```python
from build123d import *

# Parameters (mm, degrees)
F0_W     = 25
F0_H     = 25
F1_DEPTH = 50
F2_R     = 5.15
F3_DEPTH = 50.001
F5_START = -18
F4_R     = 5.15
F5_DEPTH = 32.001
F6_R     = 1
F7_SIZE  = 0.4
F8_ANGLE = 180


with BuildPart() as f1:
    # F0 (on Top) → F1 (new body)
    with BuildSketch(Plane.XY):
        Rectangle(F0_W, F0_H)
    extrude(amount=F1_DEPTH)

    # F2 (on face) → F3 (cut, through all)
    with BuildSketch(Plane.XY.offset(50)):
        Circle(F2_R)
    extrude(amount=-F3_DEPTH, mode=Mode.SUBTRACT)

    # F4 (on face) → F5 (cut)
    with BuildSketch(Plane.XY.offset(50).offset(F5_START)):
        Polygon((5.0806823689, 8.8), (-5.0806823689, 8.8), (-10.1613647377, 0), (-5.0806823689, -8.8), (5.0806823689, -8.8), (10.1613647377, 0), align=None)
        Circle(F4_R, mode=Mode.SUBTRACT)
    extrude(amount=-F5_DEPTH, mode=Mode.SUBTRACT)

    # F6
    f6_edges = [f1.edges().sort_by_distance(p)[0] for p in [
        (-12.5, 12.5, 25),
        (-12.5, -12.5, 25),
        (12.5, 12.5, 25),
        (12.5, -12.5, 25),
    ]]
    fillet(f6_edges, radius=F6_R)

    # F7
    f7_edges = [f1.edges().sort_by_distance(p)[0] for p in [
        (0, 12.5, 0),
        (12.207107, 12.207107, 0),
        (-12.207107, 12.207107, 0),
        (12.5, 0, 0),
        (-12.5, 0, 0),
        (12.207107, -12.207107, 0),
        (-12.207107, -12.207107, 0),
        (0, -12.5, 0),
        (7.621024, 4.4, 0),
        (0, 8.8, 0),
        (-7.621024, 4.4, 0),
        (-7.621024, -4.4, 0),
        (0, -8.8, 0),
        (7.621024, -4.4, 0),
        (0, 12.5, 50),
        (12.207107, 12.207107, 50),
        (-12.207107, 12.207107, 50),
        (12.5, 0, 50),
        (-12.5, 0, 50),
        (12.207107, -12.207107, 50),
        (-12.207107, -12.207107, 50),
        (0, -12.5, 50),
        (-5.15, 0, 50),
        (7.621024, 4.4, 32),
        (0, 8.8, 32),
        (-7.621024, 4.4, 32),
        (-7.621024, -4.4, 32),
        (0, -8.8, 32),
        (7.621024, -4.4, 32),
        (-5.15, 0, 32),
    ]]
    chamfer(f7_edges, length=F7_SIZE)


with BuildPart() as f1_1:
    # F8: moved
    add(f1.part.rotate(Axis((12.1, 0, 50), (0, -1, 0)), F8_ANGLE))


solid = f1_1.part
```
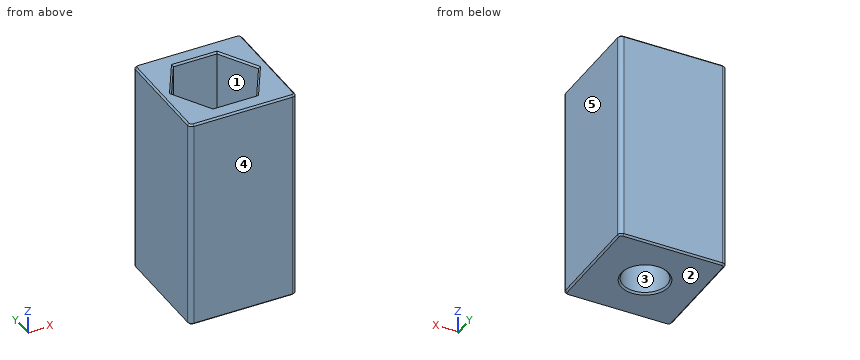
For this review, take the finished solid that the model builds, in its own axes (mm). Face numbers are marked on the shaded views. A direction names the side the tool comes from. Round coordinates to 2 decimals unless told otherwise and drop trailing zeros. Write each loop counter-clockwise with the first axis right and the second up, starting at its lowest first coordinate (ties: lowest second). Pieces come first, ordered by that corner, then holes.
1) Insertion check: pin 1 Ø5 at (x, y) = (20, 3.5) entering from +Z. The pin has a flat end and moves straight along its axis. Give the tip position at first contact, or say it passes through.
Answer below:
pin 1: stops at z = 68
2) Take a section at A-A on z = 97. Give the boundary of the cut face in (x, y).
Answer below:
outline: (11.7, -11.5) arc R1 ccw to (12.7, -12.5) - (35.7, -12.5) arc R1 ccw to (36.7, -11.5) - (36.7, 11.5) arc R1 ccw to (35.7, 12.5) - (12.7, 12.5) arc R1 ccw to (11.7, 11.5) - close; hole (14.04, 0) - (19.12, -8.8) - (29.28, -8.8) - (34.36, 0) - (29.28, 8.8) - (19.12, 8.8) - close
3) Mouldability with a two-part tool opening along Y and no side actions: class the marked faces 3, 4 and 5 as +Y half, -Y half, draft (parallel to the pull), parting line (faces both ways), or undercut.
Answer below:
face 3: undercut
face 4: -Y half
face 5: draft
4) Take a section at B-B on x = 24.2. Give the boundary of the cut face in (y, z), then the cut area to 3 significant figures.
Answer below:
outline: (-12.5, 50.4) - (-12.1, 50) - (-5.55, 50) - (-5.15, 50.4) - (-5.15, 67.6) - (-5.55, 68) - (-8.4, 68) - (-8.8, 68.4) - (-8.8, 99.6) - (-9.2, 100) - (-12.1, 100) - (-12.5, 99.6) - close; (5.15, 50.4) - (5.55, 50) - (12.1, 50) - (12.5, 50.4) - (12.5, 99.6) - (12.1, 100) - (9.2, 100) - (8.8, 99.6) - (8.8, 68.4) - (8.4, 68) - (5.55, 68) - (5.15, 67.6) - close
area: 501 mm2
5) Machinability: for the marked faces 1 and 2, which of the approach directions +Z, -Z, +X, -X, +Y, -Y give a long, thin tool a straight path to every point of the face, cutting with its end or side? Answer none if there is none.
Answer below:
face 1: +Z
face 2: -Z, +X, -X, +Y, -Y
6) For line 1 along Y through (x, z) = (24.2, 56.5); line 2 along Y through (x, z) = (25.25, 92); line 3 along Z through (x, y) = (22, -5.75), list the stretches that pass through material, from the lowest coordinate up.
Answer below:
line 1: y = -12.5 to -5.15, 5.15 to 12.5
line 2: y = -12.5 to -8.8, 8.8 to 12.5
line 3: z = 50 to 68
7) Take a section at C-C on y = 7.25. Give the boundary of the cut face in (x, z).
Answer below:
outline: (11.7, 50.4) - (12.1, 50) - (36.3, 50) - (36.7, 50.4) - (36.7, 99.6) - (36.3, 100) - (30.64, 100) - (30.18, 99.6) - (30.18, 68.4) - (29.71, 68) - (18.69, 68) - (18.22, 68.4) - (18.22, 99.6) - (17.76, 100) - (12.1, 100) - (11.7, 99.6) - close
